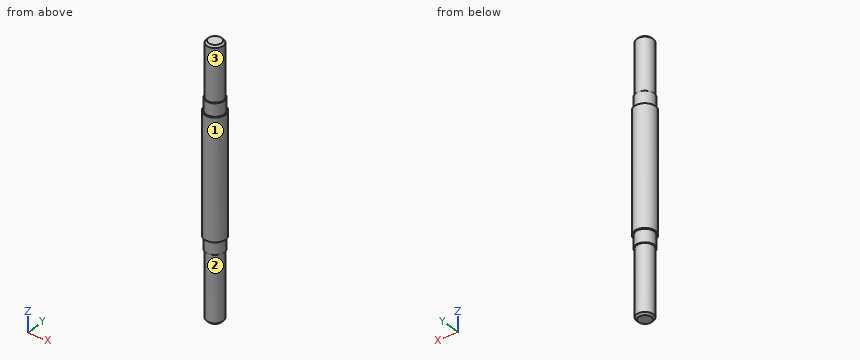
from build123d import *

# Parameters (mm, degrees)
SKETCH_R     = 5.75
PAD_DEPTH    = 65
SKETCH001_R  = 5
PAD001_DEPTH = 7
SKETCH002_R  = 4.5
PAD002_DEPTH = 29.5
SKETCH003_R  = 5
PAD003_DEPTH = 7
SKETCH004_R  = 4.5
PAD004_DEPTH = 37
CHAMFER_SIZE = 1


with BuildPart() as part:
    # Sketch → Pad (new body)
    with BuildSketch(Plane.XY):
        Circle(SKETCH_R)
    extrude(amount=PAD_DEPTH)

    # Sketch001 (on Face3 of Pad) → Pad001 (join)
    with BuildSketch(Plane.XY.offset(65)):
        Circle(SKETCH001_R)
    extrude(amount=PAD001_DEPTH)

    # Sketch002 (on Face5 of Pad001) → Pad002 (join)
    with BuildSketch(Plane.XY.offset(72)):
        Circle(SKETCH002_R)
    extrude(amount=PAD002_DEPTH)

    # Sketch003 (on Face2 of Pad002) → Pad003 (join)
    with BuildSketch(Plane(origin=(0, 0, 0), x_dir=(1, 0, 0), z_dir=(0, 0, -1))):
        Circle(SKETCH003_R)
    extrude(amount=PAD003_DEPTH)

    # Sketch004 (on Face6 of Pad003) → Pad004 (join)
    with BuildSketch(Plane(origin=(0, 0, -7), x_dir=(1, 0, 0), z_dir=(0, 0, -1))):
        Circle(SKETCH004_R)
    extrude(amount=PAD004_DEPTH)

    # Chamfer
    chamfer_edges = [part.edges().sort_by_distance(p)[0] for p in [
        (-4.5, 0, -44),
        (-4.5, 0, 101.5),
    ]]
    chamfer(chamfer_edges, length=CHAMFER_SIZE)


solid = part.part
The model under review builds one solid part; all positions refer to its coordinate system, in mm. Face numbers are marked on the shaded views. A direction names the side the tool comes from. Give positions to 0.01 mm unless a question says otherwise; leave off trailing zeros. Order: outer loops, then holes, each group sorted by start corner. A loop starts at its lowest first (then second) coordinate and runs counter-clockwise, first axis right, second up. Notation, with made-up numbers: M -17.5,-22 L 3.5,-22 A18 cw 3.5,-9 Z; hole C -6.75,73.25 d2. An arc over 180 degrees is marked long. Use one line per item in the form item = value. Start each with the question number.
Item 1: We need section D-D on z = 61. Give the boundary of the cut face in (x, y).
Item 2: We need section A-A on y = 0. Give the boundary of the cut face in (x, z), plus the area to 3 significant figures.
Item 3: Insertion check: pin 1 Ø5 at (y, z) = (3, 49) entering from -X; pin 2 Ø2 at (y, z) = (1.5, 32) entering from +X. Each pin has a flat end and moves straight along its axis. Give the tip position at first contact, or say it passes through.
Item 4: For the marked faces 1, 2 and 3, list the 3-axis set-ups (+Z, -Z, +X, -X, +Y, -Y) from which the entire face can be reached by the end or side of a thin tool; tool diameter is ignored.
Item 5: To check wall thickness, follow line 1 along Z through (x, y) = (3, 3.5); line 2 along Z through (x, y) = (-4.75, -2); line 3 along Y through (x, z) = (0, -17.5). State the ranges of each line that lie inside material, in increasing order. Write a range as from..to.
Item 6: We need section C-C on z = 83. Give the boundary of the cut face in (x, y).
Completed:
q1.outline = C 0,0 d11.5
q2.outline = M -5.75,0 L -5,0 L -5,-7 L -4.5,-7 L -4.5,-43 L -3.5,-44 L 3.5,-44 L 4.5,-43 L 4.5,-7 L 5,-7 L 5,0 L 5.75,0 L 5.75,65 L 5,65 L 5,72 L 4.5,72 L 4.5,100.5 L 3.5,101.5 L -3.5,101.5 L -4.5,100.5 L -4.5,72 L -5,72 L -5,65 L -5.75,65 Z
q2.area = 1,480 mm²
q3.pin_1 = -5.73
q3.pin_2 = 5.73
q4.face_1 = +Z, -Z
q4.face_2 = -Z
q4.face_3 = +Z
q5.line_1 = -7..72
q5.line_2 = 0..65
q5.line_3 = -4.5..4.5
q6.outline = C 0,0 d9
